Could you check a few things on this model? Use its own coordinates, in mm. Face numbers are marked on the shaded views. A direction names the side the tool comes from. Coordinates: 2 decimals unless noted, no trailing zeros. Order: outer loops, then holes, each group sorted by start corner. A loop starts at its lowest first (then second) coordinate and runs counter-clockwise, first axis right, second up. Notation, with made-up numbers: (81.25, 73) -> (107.25, 73) arc R27 ccw to (107.25, 95) -> close; hole circle Ø9 at (-2.5, 35.5). An arc over 180 degrees is marked (long way). Put each result on its own line as item: value. Start each with the question number.
Q1. Will these pins go through, and if not, where does the flat tip stop? pin 1 (4 mm diameter, centred on x = 53.5, z = -9.5, fed in from -Y); pin 2 (11.5 mm diameter, centred on x = 2, y = 14.5, fed in from +Z); pin 3 (14.5 mm diameter, centred on x = 27.5, z = -9, fed in from +Y).
Q2. Please list where these lines run through material, in increasing order: line 1 along Z through (x, y) = (0, -0.9); line 2 along Y through (x, z) = (21, -20); line 3 along Z through (x, y) = (24, 4).
Q3. If we section it at B-B (z = 0): Please give me the cut outline in (x, y), and give its area (3 significant figures).
Q4. If we section it at D-D (y = 8): Please give me the cut outline in (x, z).
Q5. If we section it at C-C (x = 17.5): Please give me the cut outline in (y, z), and give its area (3 significant figures).
Q6. For the marked faces 1 and 2, which set-ups out of +Z, -Z, +X, -X, +Y, -Y let a thin tool reach every point of the face, with its end or its side?
Q7. If we section it at A-A (x = 0): Please give me the cut outline in (y, z), and give its area (3 significant figures).
from build123d import *

# Parameters (mm, degrees)
F0_W     = 145.4322189093
F0_H     = 48
F0_R     = 14
F1_DEPTH = 2
F3_R     = 10
F4_W     = 145.4322189093
F4_H     = 25
F5_DEPTH = 2
F6_R     = 10


with BuildPart() as f1:
    # F0 (on Front) → F1 (new body)
    with BuildSketch(Plane.XZ):
        with Locations((0.9282901883, 0.5)):
            Rectangle(F0_W, F0_H)
        with Locations((-48, 0)):
            Circle(F0_R, mode=Mode.SUBTRACT)
        Circle(F0_R, mode=Mode.SUBTRACT)
        with Locations((48, 0)):
            Circle(F0_R, mode=Mode.SUBTRACT)
    extrude(amount=F1_DEPTH)

    # F3
    f3_edges = [f1.edges().sort_by_distance(p)[0] for p in [
        (73.6444, -1, 24.5),
        (-71.787819, -1, 24.5),
    ]]
    fillet(f3_edges, radius=F3_R)

    # F4 (on offset) → F5 (join)
    with BuildSketch(Plane(origin=(0, 0, -23.5), x_dir=(1, 0, 0), z_dir=(0, 0, -1))):
        with Locations((0.9282901883, -10.5)):
            Rectangle(F4_W, F4_H)
    extrude(amount=F5_DEPTH)

    # F6
    f6_edges = [f1.edges().sort_by_distance(p)[0] for p in [
        (-71.787819, 23, -24.5),
        (73.6444, 23, -24.5),
    ]]
    fillet(f6_edges, radius=F6_R)


solid = f1.part
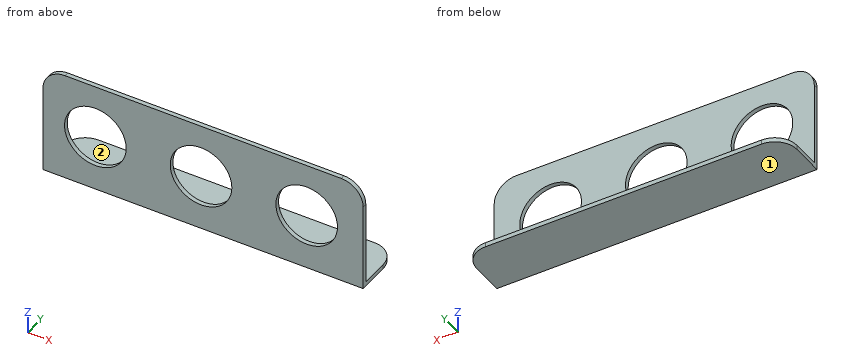
The answers:
1. pin 1: through
1. pin 2: z = -23.5
1. pin 3: y = 0
2. line 1: -25.5 to -14, 14 to 24.5
2. line 2: -2 to 0
2. line 3: -25.5 to -23.5
3. outline: (-71.79, -2) -> (-62, -2) -> (-62, 0) -> (-71.79, 0) -> close; (-34, -2) -> (-14, -2) -> (-14, 0) -> (-34, 0) -> close; (14, -2) -> (34, -2) -> (34, 0) -> (14, 0) -> close; (62, -2) -> (73.64, -2) -> (73.64, 0) -> (62, 0) -> close
3. area: 123 mm^2
4. outline: (-71.79, -25.5) -> (73.64, -25.5) -> (73.64, -23.5) -> (-71.79, -23.5) -> close
5. outline: (-2, -25.5) -> (23, -25.5) -> (23, -23.5) -> (0, -23.5) -> (0, 24.5) -> (-2, 24.5) -> close
5. area: 146 mm^2
6. face 1: -Z, +X, -X, +Y, -Y
6. face 2: +Z, +X, -X, +Y
7. outline: (-2, -25.5) -> (23, -25.5) -> (23, -23.5) -> (0, -23.5) -> (0, -14) -> (-2, -14) -> close; (-2, 14) -> (0, 14) -> (0, 24.5) -> (-2, 24.5) -> close
7. area: 90.0 mm^2
